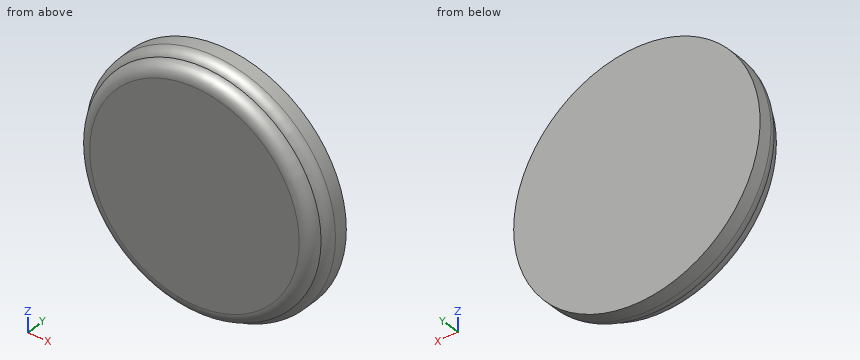
from build123d import *

# Parameters (mm, degrees)
F0_R     = 50
F1_DEPTH = 10
F2_R     = 47.5
F3_DEPTH = 5


# Not quite as in the source:
# - a fillet or chamfer that OpenCascade refuses, or shapes differently, is made with other operations: its cross-section is extruded or revolved along the edge and cut away or added


with BuildPart() as f1:
    # F0 (on Front) → F1 (new body)
    with BuildSketch(Plane.XZ):
        Circle(F0_R)
    extrude(amount=F1_DEPTH)

    # F2 (on face) → F3 (join)
    with BuildSketch(Plane.XZ.offset(10)):
        Circle(F2_R)
    extrude(amount=F3_DEPTH)

    # F4: fillet of radius 5 on 2 edges, made by hand

    # F4_s1 → F4_t2 (revolve, cut)
    with BuildSketch(Plane.XY):
        with BuildLine():
            ThreePointArc((50, -5.6698729811), (49.3301270189, -8.1698729811), (47.5, -10))
            Line((47.5, -10), (50, -10))
            Line((50, -10), (50, -5.6698729811))
        make_face()
    revolve(axis=Axis((0, -10, 0), (0, -1, 0)), mode=Mode.SUBTRACT)

    # F4_s3 → F4_t4 (revolve, cut)
    with BuildSketch(Plane.XY):
        with BuildLine():
            ThreePointArc((47.5, -10), (46.0355339059, -13.5355339059), (42.5, -15))
            Line((42.5, -15), (47.5, -15))
            Line((47.5, -15), (47.5, -10))
        make_face()
    revolve(axis=Axis((0, -15, 0), (0, -1, 0)), mode=Mode.SUBTRACT)


solid = f1.part
Verification items for the finished model (mm, model axes). Coordinates: 2 decimals unless noted, no trailing zeros. Write each loop counter-clockwise with the first axis right and the second up, starting at its lowest first coordinate (ties: lowest second). Pieces come first, ordered by that corner, then holes. Notation, with made-up numbers: (79, -17.75) - (87, -17.75) arc R13 ccw to (87, 6.25) - close; hole circle Ø11 at (62.25, 67.25). An arc over 180 degrees is marked (long way). Answer as a JSON object with one key per item and string values.
(1) Thickness scan on line 1 along Z through (x, y) = (-24, -11.75); line 2 along X through (y, z) = (-14, -36); line 3 along X through (y, z) = (-10.75, -20.5). Record the ranges inside material, lowest first.
Report:
{"line 1": "-40.62 to 40.62", "line 2": "-27.83 to 27.83", "line 3": "-42.79 to 42.79"}
(2) Cross-section at B-B on x = 0. Record the cut outline in (y, z), plus the area to 3 significant figures.
Report:
{"outline": "(-15, -42.5) arc R5 ccw to (-10, -47.5) arc R5 ccw to (-5.67, -50) - (0, -50) - (0, 50) - (-5.67, 50) arc R5 ccw to (-10, 47.5) arc R5 ccw to (-15, 42.5) - close", "area": "1,460 mm^2"}
(3) Gauge pin test, flat ends, axial feed: pin 1 Ø2 at (x, y) = (-10, -5) entering from +Z; pin 2 Ø3 at (y, z) = (-6, 22) entering from -X; pin 3 Ø2 at (x, y) = (-15, -7.5) entering from +Z. Record the tip position at first contact, or that the pin passes through.
Report:
{"pin 1": "z = 49.18", "pin 2": "x = -45.6", "pin 3": "z = 47.78"}
(4) Cross-section at A-A on z = 0. Record the cut outline in (x, y), plus the area to 3 significant figures.
Report:
{"outline": "(-50, -5.67) arc R5 ccw to (-47.5, -10) arc R5 ccw to (-42.5, -15) - (42.5, -15) arc R5 ccw to (47.5, -10) arc R5 ccw to (50, -5.67) - (50, 0) - (-50, 0) - close", "area": "1,460 mm^2"}
